For this review, use the dimensioned drawing (mm, ordinates from the lowest corner) and the shaded views. Give positions to 0.01 mm unless a question says otherwise; leave off trailing zeros. Order: outer loops, then holes, each group sorted by start corner. A loop starts at its lowest first (then second) coordinate and runs counter-clockwise, first axis right, second up.
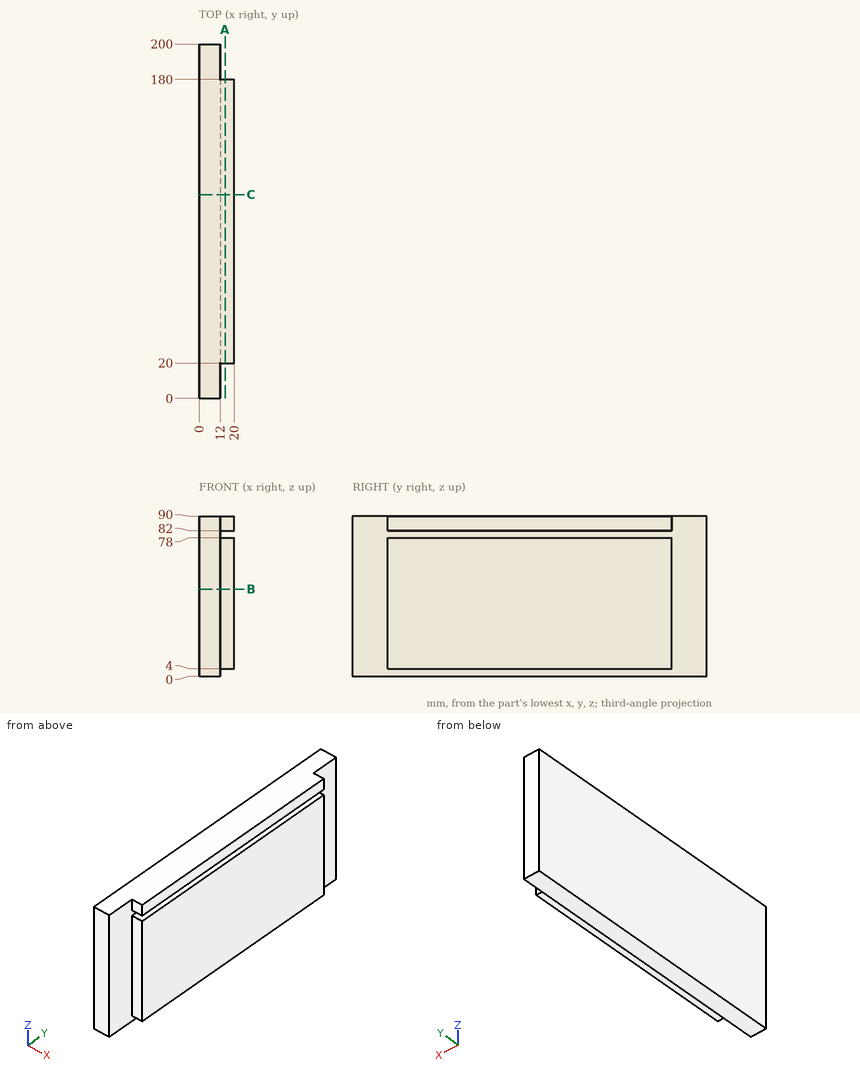
1. To check wall thickness, follow line 1 (Z direction, x = 14, y = 105); line 2 (Y direction, x = 16.25, z = 9.5); line 3 (X direction, y = 85, z = 78.5). State the ranges of each line that lie inside material, in increasing order.
2. Insertion check: pin 1 (2.5 mm diameter, centred on x = 17.5, z = 49.5, fed in from -Y); pin 2 (9 mm diameter, centred on x = 17.5, z = 85.5, fed in from +Y). Each pin has a flat end and moves straight along its axis. Give the tip position at first contact, or say it passes through.
3. Take a section at A-A (x = 14.75). Write out the cut boundary in (y, z).
4. Take a section at B-B (z = 49). Write out the cut boundary in (x, y), and give its area (3 significant figures).
5. Take a section at C-C (y = 115). Write out the cut boundary in (x, z), and give its area (3 significant figures).
Answer:
1. line 1: z = 4 to 78, 82 to 90
1. line 2: y = 20 to 180
1. line 3: x = 0 to 12
2. pin 1: stops at y = 20
2. pin 2: stops at y = 180
3. outline: (20, 4) - (180, 4) - (180, 78) - (20, 78) - close; (20, 82) - (180, 82) - (180, 90) - (20, 90) - close
4. outline: (0, 0) - (12, 0) - (12, 20) - (20, 20) - (20, 180) - (12, 180) - (12, 200) - (0, 200) - close
4. area: 3,680 mm2
5. outline: (0, 0) - (12, 0) - (12, 4) - (20, 4) - (20, 78) - (12, 78) - (12, 82) - (20, 82) - (20, 90) - (0, 90) - close
5. area: 1,740 mm2
